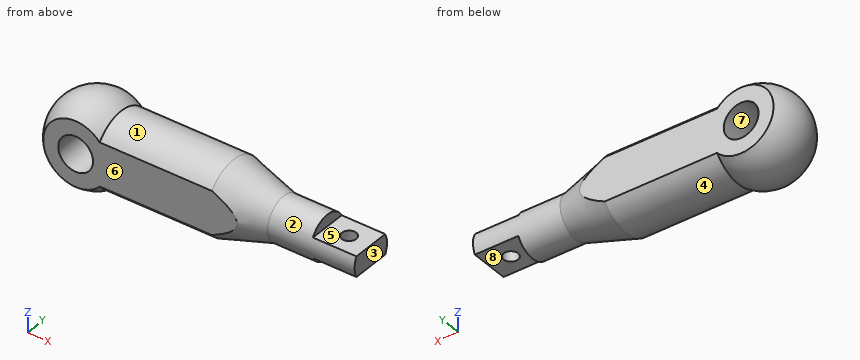
from build123d import *

# Parameters (mm, degrees)
F2_W          = 15
F2_H          = 4
F3_DEPTH      = 15.001
F3_DEPTH_BACK = 15.001
F5_DEPTH      = 109.2926164658
F6_R          = 6
F7_DEPTH      = 20.001
F8_R          = 2.5
F9_DEPTH      = 18.501


with BuildPart() as f1:
    # F0 (on Front) → F1 (revolve)
    with BuildSketch(Plane.XZ):
        with BuildLine():
            ThreePointArc((8.2915619759, 12.5), (-7.0931858273, 13.2169101843), (-15, 0))
            Line((-15, 0), (94.2916164658, 0))
            Line((94.2916164658, 0), (94.2916164658, 7.5))
            Line((94.2916164658, 7.5), (64.2916164658, 7.5))
            Line((64.2916164658, 7.5), (47, 12.5))
            Line((47, 12.5), (8.2915619759, 12.5))
        make_face()
    revolve(axis=Axis((39.6458082329, 0, 0), (-1, 0, 0)))

    # F2 (on Front) → F3 (cut, two sides)
    with BuildSketch(Plane.XZ) as f3_sk:
        with Locations((86.7916164658, 5.5)):
            Rectangle(F2_W, F2_H)
        with Locations((86.7916164658, -5.5)):
            Rectangle(F2_W, F2_H)
    extrude(amount=-F3_DEPTH, mode=Mode.SUBTRACT)
    extrude(f3_sk.sketch, amount=F3_DEPTH_BACK, mode=Mode.SUBTRACT)

    # F4 (on face) → F5 (cut, through all)
    with BuildSketch(Plane.YZ.offset(94.2916164658)):
        with BuildLine():
            ThreePointArc((10, -11.1803398875), (13.6930639376, -6.123724357), (15, 0))
            ThreePointArc((15, 0), (13.6930639376, 6.123724357), (10, 11.1803398875))
            Line((10, 11.1803398875), (10, -11.1803398875))
        make_face()
        with BuildLine():
            Line((-10, -11.1803398875), (-10, 11.1803398875))
            ThreePointArc((-10, 11.1803398875), (-15, 0), (-10, -11.1803398875))
        make_face()
    extrude(amount=-F5_DEPTH, mode=Mode.SUBTRACT)

    # F6 (on face) → F7 (cut, through all)
    with BuildSketch(Plane.XZ.offset(10)):
        Circle(F6_R)
    extrude(amount=-F7_DEPTH, mode=Mode.SUBTRACT)

    # F8 (on face) → F9 (cut, through all)
    with BuildSketch(Plane.XY.offset(3.5)):
        with Locations((86.7916164658, 0)):
            Circle(F8_R)
    extrude(amount=-F9_DEPTH, mode=Mode.SUBTRACT)


solid = f1.part
CAD build for the part. Positions are in the model's coordinates, mm. Face numbers are marked on the shaded views. A direction names the side the tool comes from. Give positions to 0.01 mm unless a question says otherwise; leave off trailing zeros. Loops run counter-clockwise (first coordinate to the right, second up) from the corner with the lowest first, then second, coordinate; pieces in that order, holes last. Notation, with made-up numbers: M -30,-22 L 22,-22 A26 ccw 22,14 Z; hole C 35,-39.75 d1. An arc over 180 degrees is marked long. Answer in a Markdown table with one row per item. Add a question column.
Item 1: Band-saw the part on B-B on y = 0. Give the cut face in (x, z).
Item 2: Band-saw the part on C-C on x = 27.5. Give the cut face in (y, z).
Item 3: Band-saw the part on D-D on x = 53. Give the cut face in (y, z).
Item 4: Probe probe 1 along Z at (x, y) = (0, 0.25); probe 2 along X at (y, z) = (3.5, -1); probe 3 along Z at (x, y) = (0, -3.25). List the from-to ranges inside material, lowest first.
Item 5: Tool access for the marked faces 1, 2, 3, 4 and 5: list every direction of +Z, -Z, +X, -X, +Y, -Y with a clear straight run to the whole face (end or side of a thin tool).
Item 6: Mould opens along Z. For the marked faces 6, 7 and 8 say: +Z half, -Z half, draft (parallel to the pull), parting line (faces both ways), or undercut.
Item 7: Band-saw the part on A-A on z = 0. Give the cut face in (x, y), then the cut area to 3 significant figures.
Item 8: Drop flat-ended pins along their axis: P1, Ø2, axis at y = 1.5, z = -6, coming from the +X side; P2, Ø8, axis at y = 4.5, z = -4, coming from the +X side; P3, Ø3, axis at x = 29.5, y = 6.5, coming from the +Z side; P4, Ø3, axis at x = 71.5, y = 8, coming from the +Z side. Give the stop position or say it passes through.
Reply:
| question | item | result |
|---|---|---|
| 1 | outline | M 8.29,-12.5 L 47,-12.5 L 64.29,-7.5 L 79.29,-7.5 L 79.29,-3.5 L 84.29,-3.5 L 84.29,3.5 L 79.29,3.5 L 79.29,7.5 L 64.29,7.5 L 47,12.5 L 8.29,12.5 A15 ccw long Z; M 89.29,-3.5 L 94.29,-3.5 L 94.29,3.5 L 89.29,3.5 Z; hole C 0,0 d12 |
| 2 | outline | M -10,-7.5 A12.5 ccw 10,-7.5 L 10,7.5 A12.5 ccw -10,7.5 Z |
| 3 | outline | M -10,-3.99 A10.77 ccw 10,-3.99 L 10,3.99 A10.77 ccw -10,3.99 Z |
| 4 | probe 1 | z = -15 to -6, 6 to 15 |
| 4 | probe 2 | x = -14.55 to -5.92, 5.92 to 94.29 |
| 4 | probe 3 | z = -14.64 to -6, 6 to 14.64 |
| 5 | face 1 | +Z, +X |
| 5 | face 2 | +X |
| 5 | face 3 | +Z, -Z, +X, +Y, -Y |
| 5 | face 4 | -Z, +X |
| 5 | face 5 | +Z, +X, +Y, -Y |
| 6 | face 6 | draft |
| 6 | face 7 | undercut |
| 6 | face 8 | -Z half |
| 7 | outline | M -11.18,-10 L -6,-10 L -6,10 L -11.18,10 A15 ccw Z; M 6,-10 L 55.65,-10 L 64.29,-7.5 L 94.29,-7.5 L 94.29,7.5 L 64.29,7.5 L 55.65,10 L 6,10 Z; hole C 86.79,0 d5 |
| 7 | area | 1,730 mm^2 |
| 8 | P1 | stops at x = 79.29 |
| 8 | P2 | stops at x = 94.29 |
| 8 | P3 | stops at z = 11.46 |
| 8 | P4 | stops at z = 3.74 |
